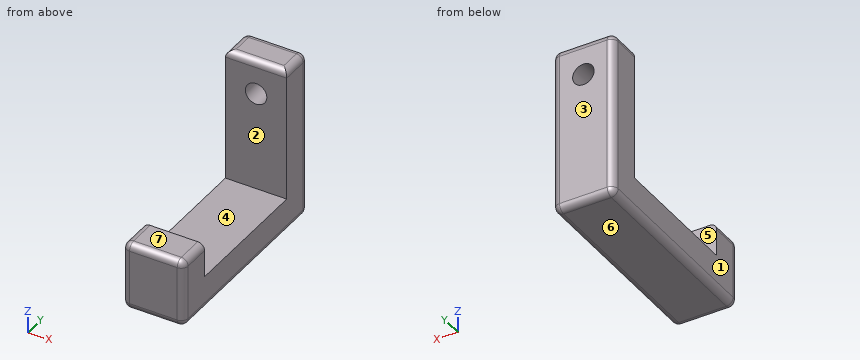
Autodesk Inventor part; units mm, degrees
ref_plane "YZ Plane" through (0, 0, 0) normal (1, 0, 0) x (0, 1, 0)
ref_plane "XZ Plane" through (0, 0, 0) normal (0, 1, 0) x (-1, 0, 0)
ref_plane "XY Plane" through (0, 0, 0) normal (0, 0, 1) x (1, 0, 0)
sketch "Sketch1" plane through (0, 0, 0) normal (1, 0, 0) x (0, 1, 0)
  line L0 (0, 0) -> (30, 0)
  line L1 (30, 0) -> (30, 24.5)
  line L2 (30, 24.5) -> (25, 24.5)
  line L3 (25, 24.5) -> (25, 5)
  line L4 (25, 5) -> (5, 5)
  line L5 (5, 5) -> (5, 10)
  line L6 (5, 10) -> (0, 10)
  line L7 (0, 10) -> (0, 0)
  line L8 (25, 5) -> (32.5, 5) construction
  dimension "d0" = 30
  dimension "d1" = 24.5
  dimension "d2" = 5
  dimension "d3" = 19.5
  dimension "d9" = 5
  dimension "d10" = 5
extrude "Extrusion1" add sketch "Sketch1" along normal blind 9
sketch "Sketch4" plane through (0, 30, 24.5) normal (0, 1, 0) x (1, 0, 0)
  circle A0 centre (4.5, 5) radius 1.575
  line L0 (0, 0) -> (9, 0)
  line L1 (0, 24.5) -> (0, 0)
  dimension "d18" = 3.15
  dimension "d19" = 5
  dimension "d20" = 4.5
extrude "Extrusion3" cut sketch "Sketch4" against normal blind 5
fillet "Fillet1" radius 1 15 edges at (9, 0, 5) (4.5, 0, 10) (0, 0, 5) (4.5, 0, 0) (9, 15, 0) (0, 15, 0) (9, 30, 12.25) (4.5, 30, 0) (0, 30, 12.25) (4.5, 30, 24.5) (4.5, 25, 24.5) (9, 27.5, 24.5) (0, 27.5, 24.5) (9, 2.5, 10) (0, 2.5, 10)
properties part number "bed_spring_holder_front" material "Plastic, Opaque Black"
Here's how the part is built. I have some questions about the finished solid (model axes, mm). Face numbers are marked on the shaded views. A direction names the side the tool comes from. Give positions to 0.01 mm unless a question says otherwise; leave off trailing zeros. Write each loop counter-clockwise with the first axis right and the second up, starting at its lowest first coordinate (ties: lowest second). Pieces come first, ordered by that corner, then holes.
(1) Will these pins go through, and if not, where does the flat tip stop? pin 1 (2.5 mm diameter, centred on x = 3.5, z = 18, fed in from -Y); pin 2 (1.2 mm diameter, centred on x = 4, y = 3.5, fed in from +Z); pin 3 (1.9 mm diameter, centred on x = 4.5, z = 19.5, fed in from +Y); pin 4 (4.5 mm diameter, centred on x = 6, y = 16.5, fed in from +Z).
Output values:
pin 1: stops at y = 25
pin 2: stops at z = 10
pin 3: passes through
pin 4: stops at z = 5
(2) If I drill on L1, parallel to X at y = 26.95, z = 19.5 (3 decimals); L2, parallel to Y at x = 1, z = 19.25; L3, parallel to Z at x = 7.25, y = 3, over which ranges is the centre line in solid material (lowest first)?
Output values:
L1: x = 0 to 2.925, 6.075 to 9
L2: y = 25 to 30
L3: z = 0 to 10
(3) Imagine slicing it at D-D, the plane z = 19.5. Write out the boundary of the cut face in (x, y) (3 decimals), and give its area (3 significant figures).
Output values:
outline: (0, 25) - (2.925, 25) - (2.925, 30) - (1, 30) arc R1 ccw to (0, 29) - close; (6.075, 25) - (9, 25) - (9, 29) arc R1 ccw to (8, 30) - (6.075, 30) - close
area: 28.8 mm2
(4) Imagine slicing it at C-C, the plane x = 2.5. Write out the boundary of the cut face in (y, z).
Output values:
outline: (0, 1) arc R1 ccw to (1, 0) - (29, 0) arc R1 ccw to (30, 1) - (30, 23.5) arc R1 ccw to (29, 24.5) - (26, 24.5) arc R1 ccw to (25, 23.5) - (25, 5) - (5, 5) - (5, 10) - (1, 10) arc R1 ccw to (0, 9) - close
(5) Imagine slicing it at A-A, the plane z = 8.5. Write out the boundary of the cut face in (x, y), and give its area (3 significant figures).
Output values:
outline: (0, 1) arc R1 ccw to (1, 0) - (8, 0) arc R1 ccw to (9, 1) - (9, 5) - (0, 5) - close; (0, 25) - (9, 25) - (9, 29) arc R1 ccw to (8, 30) - (1, 30) arc R1 ccw to (0, 29) - close
area: 89.1 mm2
(6) Imagine slicing it at B-B, the plane x = 4.5. Write out the boundary of the cut face in (y, z) (3 decimals).
Output values:
outline: (0, 1) arc R1 ccw to (1, 0) - (29, 0) arc R1 ccw to (30, 1) - (30, 17.925) - (25, 17.925) - (25, 5) - (5, 5) - (5, 10) - (1, 10) arc R1 ccw to (0, 9) - close; (25, 21.075) - (30, 21.075) - (30, 23.5) arc R1 ccw to (29, 24.5) - (26, 24.5) arc R1 ccw to (25, 23.5) - close
(7) Thinking about a two-plate mould opening in Y: for the marked faces 1, 2, 3 and 4, which applies, pulls with the +Y half, pulls with the -Y half, needs draft (parallel to the pull), parting line crosses it, or undercut?
Output values:
face 1: needs draft
face 2: undercut
face 3: pulls with the +Y half
face 4: undercut
(8) On a 3-axis mill with a long thin cutter (end or side, diameter ignored), from which of +Z, -Z, +X, -X, +Y, -Y can I reach the whole of each face in a straight line? I mean the marked faces 5, 6 and 7. Say none if no direction works.
Output values:
face 5: +Z, +X, -X
face 6: -Z, +X, -X, +Y, -Y
face 7: +Z, +X, -X, -Y
